For this review, take the finished solid that the model builds, in its own axes (mm). Face numbers are marked on the shaded views. Coordinates: 2 decimals unless noted, no trailing zeros. Write each loop counter-clockwise with the first axis right and the second up, starting at its lowest first coordinate (ties: lowest second). Pieces come first, ordered by that corner, then holes.
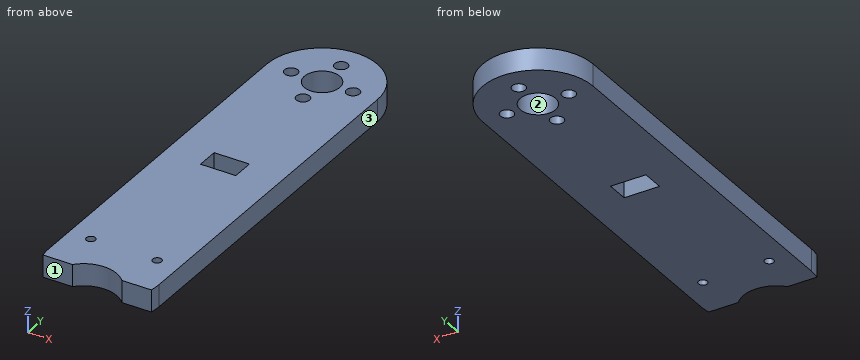
```python
from build123d import *

# Parameters (mm, degrees)
SKETCH1_R           = 1
SKETCH1_R_2         = 1.5
SKETCH1_R_3         = 4
BOSS_EXTRUDE2_DEPTH = 5
SKETCH2_W           = 8
SKETCH2_H           = 5
CUT_EXTRUDE1_DEPTH  = 10


with BuildPart() as part:
    # Sketch1 → Boss-Extrude2 (new body)
    with BuildSketch(Plane.XY):
        with BuildLine():
            Line((-12.5, 40), (-12.5, -40))
            ThreePointArc((-12.5, -40), (-12.436701913, -41.256362025), (-12.247448714, -42.5))
            Line((-12.247448714, -42.5), (-5.590169944, -42.5))
            ThreePointArc((-5.590169944, -42.5), (0, -40), (5.590169944, -42.5))
            Line((5.590169944, -42.5), (12.247448714, -42.5))
            ThreePointArc((12.247448714, -42.5), (12.436701913, -41.256362025), (12.5, -40))
            Line((12.5, -40), (12.5, 40))
            ThreePointArc((12.5, 40), (0, 52.5), (-12.5, 40))
        make_face()
        with Locations((-7.5, -32.65)):
            Circle(SKETCH1_R, mode=Mode.SUBTRACT)
        with Locations((7.5, -32.65)):
            Circle(SKETCH1_R, mode=Mode.SUBTRACT)
        with Locations((-7, 40)):
            Circle(SKETCH1_R_2, mode=Mode.SUBTRACT)
        with Locations((0, 40)):
            Circle(SKETCH1_R_3, mode=Mode.SUBTRACT)
        with Locations((0, 33)):
            Circle(SKETCH1_R_2, mode=Mode.SUBTRACT)
        with Locations((0, 47)):
            Circle(SKETCH1_R_2, mode=Mode.SUBTRACT)
        with Locations((7, 40)):
            Circle(SKETCH1_R_2, mode=Mode.SUBTRACT)
    extrude(amount=BOSS_EXTRUDE2_DEPTH)

    # Sketch2 → Cut-Extrude1 (cut)
    with BuildSketch(Plane.XY.offset(6)):
        with Locations((0, 4.38)):
            Rectangle(SKETCH2_W, SKETCH2_H)
    extrude(amount=-CUT_EXTRUDE1_DEPTH, mode=Mode.SUBTRACT)


solid = part.part
```
Q1. Add section B-B (z = 0.95). Give the number of separate pieces and of enclosed holes in the cut face, then the cut area to 3 significant figures.
Ans:
separate pieces: 1
enclosed holes: 8
area: 2,160 mm2
Q2. Add section D-D (y = 33). State the section outline as (x, z) points.
Ans:
outline: (-12.5, 0) - (-1.5, 0) - (-1.5, 5) - (-12.5, 5) - close; (1.5, 0) - (12.5, 0) - (12.5, 5) - (1.5, 5) - close
Q3. Clearance check with flat-ended pins moving along their axes: pin 1 Ø3 at (x, y) = (-2, 14) entering from -Z; pin 2 Ø2.5 at (x, y) = (7, 40) entering from +Z; pin 3 Ø2 at (x, z) = (3, 3) entering from +Y; pin 4 Ø2.5 at (x, z) = (-1, 1.5) entering from -Y. State where each tip first meets the part, or that it passes through.
Ans:
pin 1: stops at z = 0
pin 2: passes through
pin 3: stops at y = 52.34
pin 4: stops at y = -40.35
Q4. Draft analysis for pull direction X (two halves, no side actions). For the marked faces 1, 2 and 3, state which applies: +X half, -X half, draft (parallel to the pull), parting line (faces both ways), or undercut.
Ans:
face 1: draft
face 2: undercut
face 3: +X half
Q5. Add section A-A (y = 4). State the section outline as (x, z) points.
Ans:
outline: (-12.5, 0) - (-4, 0) - (-4, 5) - (-12.5, 5) - close; (4, 0) - (12.5, 0) - (12.5, 5) - (4, 5) - close
Q6. For probe 1 along Y at (x, z) = (0, 2); probe 2 along Y at (x, z) = (1, 0.35); probe 3 along Y at (x, z) = (-3, 0.9), list the stretches that pass through material, from the lowest coordinate up.
Ans:
probe 1: y = -40 to 1.88, 6.88 to 31.5, 34.5 to 36, 44 to 45.5, 48.5 to 52.5
probe 2: y = -40.07 to 1.88, 6.88 to 31.88, 34.12 to 36.13, 43.87 to 45.88, 48.12 to 52.46
probe 3: y = -40.63 to 1.88, 6.88 to 37.35, 42.65 to 52.13
Q7. Add section C-C (y = -32.65). State the section outline as (x, z) points.
Ans:
outline: (-12.5, 0) - (-8.5, 0) - (-8.5, 5) - (-12.5, 5) - close; (-6.5, 0) - (6.5, 0) - (6.5, 5) - (-6.5, 5) - close; (8.5, 0) - (12.5, 0) - (12.5, 5) - (8.5, 5) - close
